The model under review builds one solid part; all positions refer to its coordinate system, in mm. A direction names the side the tool comes from. Round coordinates to 2 decimals unless told otherwise and drop trailing zeros. Write each loop counter-clockwise with the first axis right and the second up, starting at its lowest first coordinate (ties: lowest second). Pieces come first, ordered by that corner, then holes. Notation, with made-up numbers: (-30, 21) -> (26, 21) arc R11 ccw to (26, 27) -> close; hole circle Ø10 at (-19.75, 37). An arc over 180 degrees is marked (long way). Answer as a JSON object with one key per item and string values. Group by question number.
1) To check wall thickness, follow probe 1 along Z at (x, y) = (-26, 9); probe 2 along Y at (x, z) = (0, 18.25); probe 3 along X at (y, z) = (10.5, 11.25). State the ranges of each line that lie inside material, in increasing order. Write a range as [from, to].
2) We need section A-A, the plane y = 9.5. Write out the cut boundary in (x, z), then the cut area to 3 significant figures.
3) Insertion check: pin 1 Ø12 at (y, z) = (30, 5.5) entering from +X; pin 2 Ø7 at (x, z) = (26, 12) entering from -Y; pin 3 Ø5.5 at (y, z) = (25, 6.5) entering from -X; pin 4 Ø8 at (x, y) = (-26.5, 19) entering from -Z. Each pin has a flat end and moves straight along its axis. Give the tip position at first contact, or say it passes through.
4) Mouldability with a two-part tool opening along X and no side actions: class faces 1 (the flat face through (-18, 29, 12)), 2 (the flat face through (-8, 7, 0)), 3 (the cylindrical face through (6.5, 8.3, 11.8)), 4 (the cylindrical face through (21.504, 9.988, 11.802)) as pulls with the +X half, pulls with the -X half, needs draft (parallel to the pull), parting line crosses it, or undercut.
5) We need section C-C, the plane x = 0. Write out the cut boundary in (y, z), then the cut area to 3 significant figures.
6) We need section D-D, the plane y = 20.7. Write out the cut boundary in (x, z).
7) Machinability: for faces 5 (the flat face through (30, 19.7, 9)), 6 (the flat face through (0, 0, 12)), 7 (the flat face through (-30, 19.7, 9)), which of the approach directions +Z, -Z, +X, -X, +Y, -Y give a long, thin tool a straight path to every point of the face, cutting with its end or side? Answer none if there is none.
8) We need section B-B, the plane z = 12. Write out the cut boundary in (x, y).
from build123d import *

# Parameters (mm, degrees)
ESBO_O1_R                = 14
RESSALTO_EXTRUS_O3_DEPTH = 24
SKETCH2_R                = 4.5
CUT_EXTRUDE1_DEPTH       = 47.787712062


with BuildPart() as part:
    # Esboço1 → Ressalto-extrusão3 (new body)
    with BuildSketch(Plane.XY):
        Polygon((-35, 0), (35, 0), (35, 19.7), (18, 19.7), (18, 38.7), (-18, 38.7), (-18, 19.7), (-35, 19.7), align=None)
        with Locations((0, 20.7)):
            Circle(ESBO_O1_R, mode=Mode.SUBTRACT)
    extrude(amount=RESSALTO_EXTRUS_O3_DEPTH)

    # Sketch2 → Cut-Extrude1 (cut, through all)
    with BuildSketch(Plane(origin=(0, 19.7, 0), x_dir=(1, 0, 0), z_dir=(0, 1, 0))):
        with Locations(Location((-26, -12, 0), (0, 0, 180))):
            Circle(SKETCH2_R)
        with Locations((26, -12)):
            Circle(SKETCH2_R)
    extrude(amount=-CUT_EXTRUDE1_DEPTH, mode=Mode.SUBTRACT)


solid = part.part
Here are the results:
{
 "1": {"probe 1": "z = [0, 7.5], [16.5, 24]", "probe 2": "y = [0, 6.7], [34.7, 38.7]", "probe 3": "x = [-35, -30.44], [-21.56, -9.59], [9.59, 21.56], [30.44, 35]"},
 "2": {"outline": "(-35, 0) -> (-8.4, 0) -> (-8.4, 24) -> (-35, 24) -> close; (8.4, 0) -> (35, 0) -> (35, 24) -> (8.4, 24) -> close; hole circle Ø9 at (-26, 12); hole circle Ø9 at (26, 12)", "area": "1,150 mm^2"},
 "3": {"pin 1": "stops at x = 18", "pin 2": "passes through", "pin 3": "stops at x = -18", "pin 4": "stops at z = 0"},
 "4": {"face 1": "pulls with the -X half", "face 2": "needs draft", "face 3": "undercut", "face 4": "undercut"},
 "5": {"outline": "(0, 0) -> (6.7, 0) -> (6.7, 24) -> (0, 24) -> close; (34.7, 0) -> (38.7, 0) -> (38.7, 24) -> (34.7, 24) -> close", "area": "257 mm^2"},
 "6": {"outline": "(-18, 0) -> (-14, 0) -> (-14, 24) -> (-18, 24) -> close; (14, 0) -> (18, 0) -> (18, 24) -> (14, 24) -> close"},
 "7": {"face 5": "+Z, -Z, +X, +Y", "face 6": "+Z, -Z, +X, -X, -Y", "face 7": "+Z, -Z, -X, +Y"},
 "8": {"outline": "(-35, 0) -> (-30.5, 0) -> (-30.5, 19.7) -> (-35, 19.7) -> close; (-21.5, 0) -> (21.5, 0) -> (21.5, 19.7) -> (18, 19.7) -> (18, 38.7) -> (-18, 38.7) -> (-18, 19.7) -> (-21.5, 19.7) -> close; (30.5, 0) -> (35, 0) -> (35, 19.7) -> (30.5, 19.7) -> close; hole circle Ø28 at (0, 20.7)"}
}
